Job drawing, mm, ordinate dimensions from the low corner. One solid piece. Give positions to 0.01 mm unless a question says otherwise; leave off trailing zeros. Write each loop counter-clockwise with the first axis right and the second up, starting at its lowest first coordinate (ties: lowest second). Pieces come first, ordered by that corner, then holes. Notation, with made-up numbers: M -18,1 L 40,1 A36 ccw 40,40 Z; hole C -3.5,86 d3. An arc over 180 degrees is marked long. Use CSV: the item, a comma, the result in double quotes. Start each with the question number.
Item 1: Cut at B-B (z = 5). List the corners of the cut face in (x, y), then the cut area to 3 significant figures.
Item 2: Mould opens along X. For the marked faces 1, 2 and 3 say: released by +X, released by -X, zero draft, split by the parting line, or undercut.
Item 3: Cut at C-C (y = 6.5). Count the separate pieces of the cut face and the enclosed holes in it, then the cut area to 3 significant figures.
Item 4: Cut at D-D (z = 37.5). List the corners of the cut face in (x, y), then the cut area to 4 significant figures.
Item 5: Pin check, flat tips, straight feed: pin 1 (11 mm diameter, centred on x = 91, z = 37.5, fed in from -Y); pin 2 (8 mm diameter, centred on y = 9, z = 35, fed in from -X). Stop position of each tip, or through.
Item 6: Cut at A-A (x = 91). List the corners of the cut face in (y, z), then the cut area to 3 significant figures.
Item 7: Drill centre lines: line 1 (Z direction, x = 14, y = 8); line 2 (Z direction, x = 75, y = 8.75); line 3 (X direction, y = 9.25, z = 12). Where is each one in solid material? Low to high. Write a range as [from, to].
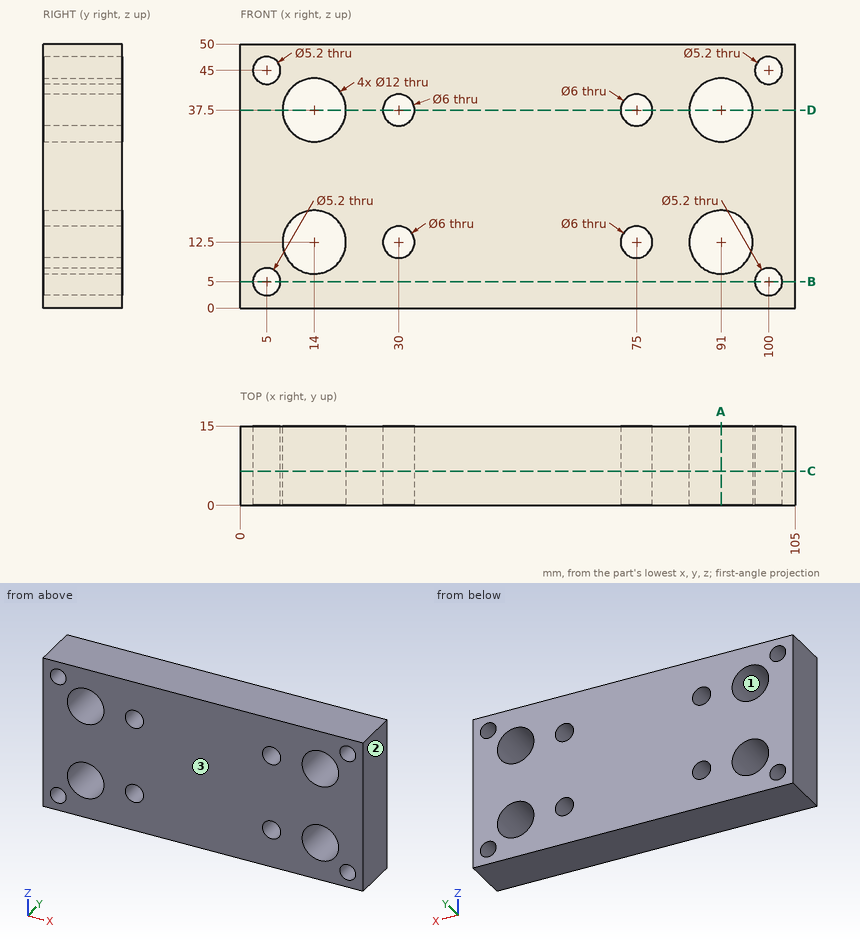
Worked answers:
1,outline,"M 0,0 L 2.4,0 L 2.4,15 L 0,15 Z; M 7.6,0 L 97.4,0 L 97.4,15 L 7.6,15 Z; M 102.6,0 L 105,0 L 105,15 L 102.6,15 Z"
1,area,"1,420 mm^2"
2,face 1,"undercut"
2,face 2,"released by +X"
2,face 3,"zero draft"
3,separate pieces,"1"
3,enclosed holes,"12"
3,area,"4,600 mm^2"
4,outline,"M 0,0 L 8,0 L 8,15 L 0,15 Z; M 20,0 L 27,0 L 27,15 L 20,15 Z; M 33,0 L 72,0 L 72,15 L 33,15 Z; M 78,0 L 85,0 L 85,15 L 78,15 Z; M 97,0 L 105,0 L 105,15 L 97,15 Z"
4,area,"1,035 mm^2"
5,pin 1,"passes through"
5,pin 2,"stops at x = 0"
6,outline,"M 0,0 L 15,0 L 15,6.5 L 0,6.5 Z; M 0,18.5 L 15,18.5 L 15,31.5 L 0,31.5 Z; M 0,43.5 L 15,43.5 L 15,50 L 0,50 Z"
6,area,"390 mm^2"
7,line 1,"z = [0, 6.5], [18.5, 31.5], [43.5, 50]"
7,line 2,"z = [0, 9.5], [15.5, 34.5], [40.5, 50]"
7,line 3,"x = [0, 8.02], [19.98, 27.04], [32.96, 72.04], [77.96, 85.02], [96.98, 105]"
